Verification items for the finished model (mm, model axes). Face numbers are marked on the shaded views. Give positions to 0.01 mm unless a question says otherwise; leave off trailing zeros. Answer as CSV lines item,"result".
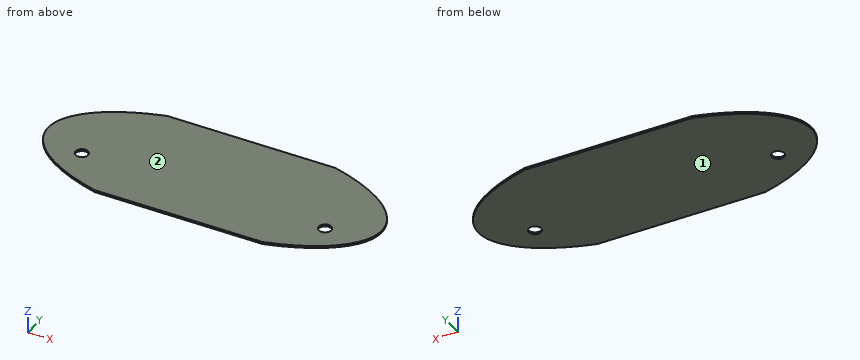
```python
from build123d import *

# Parameters (mm, degrees)
SKETCH1_RX          = 240
SKETCH1_RY          = 110
BOSS_EXTRUDE1_DEPTH = 3
SKETCH12_R          = 9
CUT_EXTRUDE8_DEPTH  = 265.024620064
SKETCH13_W          = 480
SKETCH13_H          = 15
CUT_EXTRUDE9_DEPTH  = 265.024620064


with BuildPart() as part:
    # Sketch1 → Boss-Extrude1 (new body)
    with BuildSketch(Plane.XY):
        with Locations((0, 0)):
            Ellipse(SKETCH1_RX, SKETCH1_RY)
    extrude(amount=-BOSS_EXTRUDE1_DEPTH)

    # Sketch12 → Cut-Extrude8 (cut, through all)
    with BuildSketch(Plane.XY):
        with Locations((175, -30)):
            Circle(SKETCH12_R)
        with Locations(Location((-175, -30, 0), (0, 0, 180))):
            Circle(SKETCH12_R)
    extrude(amount=-CUT_EXTRUDE8_DEPTH, mode=Mode.SUBTRACT)

    # Sketch13 → Cut-Extrude9 (cut, through all)
    with BuildSketch(Plane.XY):
        with Locations((0, -102.5)):
            Rectangle(SKETCH13_W, SKETCH13_H)
        with Locations((0, 102.5)):
            Rectangle(SKETCH13_W, SKETCH13_H)
    extrude(amount=-CUT_EXTRUDE9_DEPTH, mode=Mode.SUBTRACT)


solid = part.part
```
1) Draft check along Z on the marked faces 1 and 2. Enter one of: +Z half, -Z half, draft (parallel to the pull), parting line (faces both ways), or undercut.
Reported:
face 1,"-Z half"
face 2,"+Z half"
2) Depth check by flat-ended pin: pin 1 (10 mm diameter, centred on x = -145.5, y = 69, fed in from +Z); pin 2 (1 mm diameter, centred on y = 12, z = -1, fed in from -X). Enter the tip coordinate at first touch or a pass-through.
Reported:
pin 1,"z = 0"
pin 2,"x = -238.68"
3) Section check A-A (z = -1.95). State how many separate pieces and enclosed holes the cut face has, and give its area (3 significant figures).
Reported:
separate pieces,"1"
enclosed holes,"2"
area,"77,500 mm²"
4) Scan lines: line 1 along X through (y, z) = (-30.5, -0.55); line 2 along Y through (x, z) = (175, -1); line 3 along Y through (x, z) = (-159, -1.65). Record each from-to range of solid material in increasing order.
Reported:
line 1,"-230.59 to -183.99, -166.01 to 166.01, 183.99 to 230.59"
line 2,"-75.28 to -39, -21 to 75.28"
line 3,"-82.4 to 82.4"
